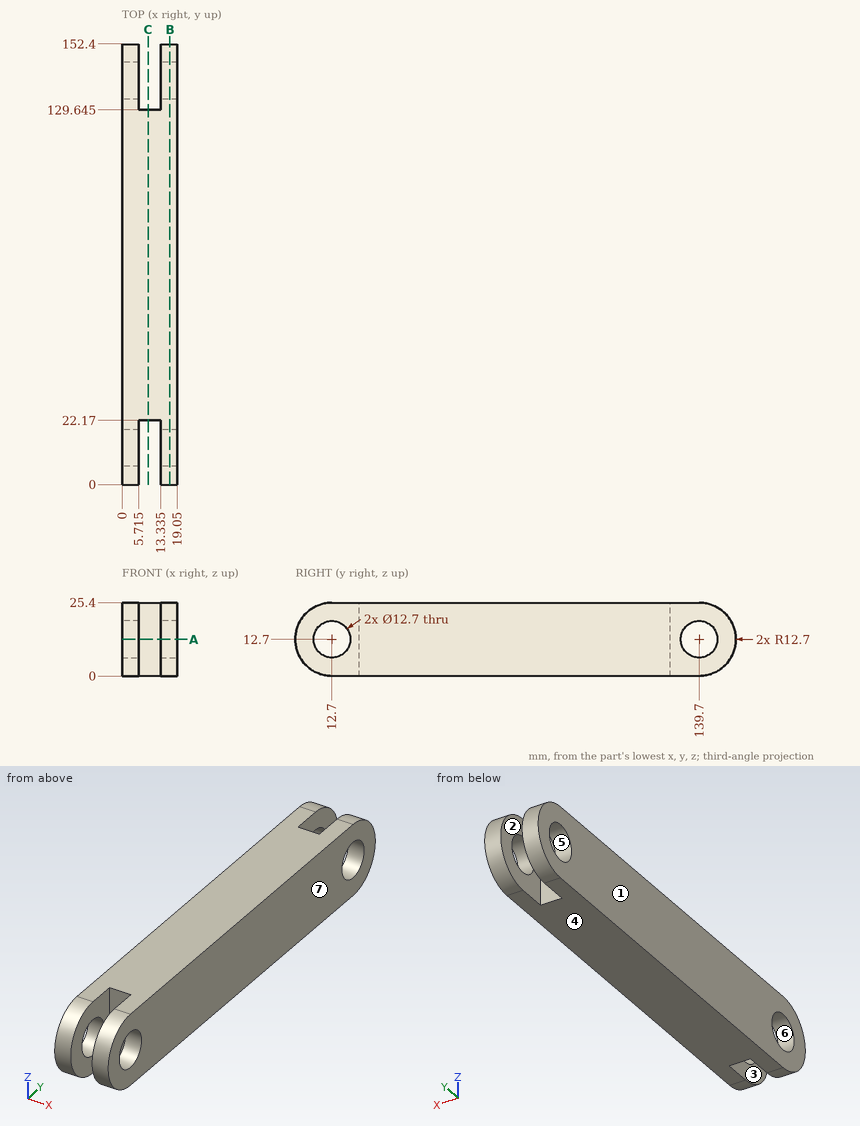
Geometry check sheet. Reference: drawing and pictorial views, mm from the part's lowest x, y, z. A direction names the side the tool comes from. Coordinates: 2 decimals unless noted, no trailing zeros. Order: outer loops, then holes, each group sorted by start corner. A loop starts at its lowest first (then second) coordinate and runs counter-clockwise, first axis right, second up. Notation, with made-up numbers: (14, 33.5) -> (22, 33.5) arc R14 ccw to (22, 54.5) -> close; hole circle Ø2 at (-30, 47.25). An arc over 180 degrees is marked (long way). Write item = value, one per line. Start each with the question number.
1) Cross-section at A-A (z = 12.7). State how many separate pieces and enclosed holes the cut face has, then the cut area to 3 significant figures.
2) Material ranges on L1, parallel to Y at x = 4.5, z = 12.75; L2, parallel to Z at x = 16.3, y = 12.7; L3, parallel to Y at x = 5, z = 10, recorded low to high.
3) Go/stop test with flat-tipped pins: P1, Ø8, axis at x = 7.5, z = 18, coming from the +Y side; P2, Ø6, axis at x = 10, z = 17, coming from the -Y side; P3, Ø8, axis at x = 12.5, z = 5.5, coming from the -Y side. Record where each tip stops, or that it passes through.
4) Cross-section at B-B (x = 16.5). Enter the section's corners in (y, z), then the cut area to 3 significant figures.
5) Mould release check, pull along Z, two halves, no side actions. Record for the marked faces 4, 5, 6 and 7: +Z half, -Z half, draft (parallel to the pull), parting line (faces both ways), or undercut.
6) Cross-section at C-C (x = 9). Enter the section's corners in (y, z) (1 decimal), then the cut area to 3 significant figures.
7) Access from +Z, -Z, +X, -X, +Y, -Y to the whole of each face (thin tool, end or side, straight path). Record for the marked faces 1, 2 and 3.
Ans:
q1.separate_pieces = 5
q1.enclosed_holes = 0
q1.area = 2,270 mm²
q2.L1 = 0 to 6.35, 19.05 to 133.35, 146.05 to 152.4
q2.L2 = 0 to 6.35, 19.05 to 25.4
q2.L3 = 0.29 to 6.95, 18.45 to 133.95, 145.45 to 152.11
q3.P1 = 152.28
q3.P2 = 22.17
q3.P3 = 0.43
q4.outline = (12.7, 0) -> (139.7, 0) arc R12.7 ccw to (139.7, 25.4) -> (12.7, 25.4) arc R12.7 ccw to start; hole circle Ø12.7 at (12.7, 12.7); hole circle Ø12.7 at (139.7, 12.7)
q4.area = 3,480 mm²
q5.face_4 = -Z half
q5.face_5 = undercut
q5.face_6 = undercut
q5.face_7 = draft
q6.outline = (22.2, 0) -> (129.6, 0) -> (129.6, 25.4) -> (22.2, 25.4) -> close
q6.area = 2,730 mm²
q7.face_1 = +Z, -Z, -X, +Y, -Y
q7.face_2 = +Z, -Z, +Y
q7.face_3 = +Z, -Z, -Y
